Geometry: final body of the model. Coordinates: model frame, mm. A direction names the side the tool comes from. Round coordinates to 2 decimals unless told otherwise and drop trailing zeros. Write each loop counter-clockwise with the first axis right and the second up, starting at its lowest first coordinate (ties: lowest second). Pieces come first, ordered by that corner, then holes. Notation, with made-up numbers: (26, -7.75) -> (72, -7.75) arc R14 cw to (72, 1.25) -> close; hole circle Ø8 at (-6.5, 17). An arc over 180 degrees is marked (long way). One line per item, written item: value. Start each with the question number.
from build123d import *

# Parameters (mm, degrees)
SKETCH_1_W               = 56
SKETCH_1_H               = 30
EXTRUDE_1_DEPTH          = 8
SKETCH_3_W               = 32
SKETCH_3_H               = 30
EXTRUDE_2_DEPTH          = 4
EXTRUDE_3_DEPTH          = 12
EXTRUDE_4_DEPTH          = 8
CUT_EXTRUDE_1_DEPTH      = 46.803929962
CUT_EXTRUDE_1_DEPTH_BACK = 46.803929962


with BuildPart() as part:
    # Sketch 1 → Extrude 1 (new body)
    with BuildSketch(Plane(origin=(0, 0, 0), x_dir=(1, 0, 0), z_dir=(0, 1, 0))):
        Rectangle(SKETCH_1_W, SKETCH_1_H)
    extrude(amount=EXTRUDE_1_DEPTH)

    # Sketch 3 → Extrude 2 (add)
    with BuildSketch(Plane(origin=(0, 8, 0), x_dir=(1, 0, 0), z_dir=(0, 1, 0))):
        with Locations((-12, 0)):
            Rectangle(SKETCH_3_W, SKETCH_3_H)
    extrude(amount=EXTRUDE_2_DEPTH)

    # Sketch 7 → Extrude 3 (add)
    with BuildSketch(Plane.XY.offset(-15)):
        with BuildLine():
            Line((28, 8), (28, 21))
            ThreePointArc((28, 21), (16, 33), (4, 21))
            Line((4, 21), (4, 8))
            Line((4, 8), (28, 8))
        make_face()
        with BuildLine():
            ThreePointArc((10, 16), (16, 10), (22, 16))
            Line((22, 16), (22, 21))
            ThreePointArc((22, 21), (16, 27), (10, 21))
            Line((10, 21), (10, 16))
        make_face(mode=Mode.SUBTRACT)
    extrude(amount=EXTRUDE_3_DEPTH)

    # Sketch 7_4 → Extrude 4 (add)
    with BuildSketch(Plane.XY.offset(-15)):
        with BuildLine():
            Line((-28, 22.220866923), (-28, 12))
            Line((-28, 12), (4, 12))
            Line((4, 12), (4, 21))
            ThreePointArc((4, 21), (6.528997501, 28.368860948), (13.050018612, 32.631750075))
            Line((13.050018612, 32.631750075), (-28, 22.220866923))
        make_face()
    extrude(amount=EXTRUDE_4_DEPTH)

    # Sketch 13 → Cut-Extrude 1 (cut, two sides: drawn at the far end of the back side and taken through both)
    with BuildSketch(Plane(origin=(0, 0, 0), x_dir=(0, 0, -1), z_dir=(1, 0, 0)).offset(-CUT_EXTRUDE_1_DEPTH_BACK)):
        Polygon((0, 0), (6, 0), (8.886751346, 5), (-8.886751346, 5), (-6, 0), align=None)
    extrude(amount=CUT_EXTRUDE_1_DEPTH + CUT_EXTRUDE_1_DEPTH_BACK, mode=Mode.SUBTRACT)


solid = part.part
(1) Line query: probe 1 along Y at (x, z) = (9, 12); probe 2 along Y at (x, z) = (3.5, -2.25); probe 3 along Z at (x, y) = (-10.5, 17). Output: solid intervals per line, ascending.
(2) Set-up query: faces 5 (the face through (-12, 12, 4)), 6 (the face through (20.351, 32.183, -7.751)), 7 (the face through (10, 19, -9)), 8 (the face through (-7.19, 27.5, -11.06)), 9 (the face through (10, 23, -3)). Return all of +Z, -Z, +X, -X, +Y, -Y with unobstructed straight access to the full face (end or side cutting, diameter ignored); none if empty.
(3) Pull-direction query (Y, two-part tool) for faces 1 (the face through (-28, 9, -4)), 2 (the face through (16, 8, 6)), 3 (the face through (-0.392, 2.465, -7.423)), 4 (the face through (-0.39, 2.53, 7.46)); classes: pulls with the +Y half, pulls with the -Y half, needs draft (parallel to the pull), parting line crosses it, or undercut.
(4) Section query D-D (y = 30). Output: boundary loops of the cut face in (x, z), and give its area (3 significant figures).
(5) Section query C-C (x = -17.5). Output: boundary loops of the cut face in (y, z), and give its area (3 significant figures).
(6) Pin query (flat end, axial travel): pin 1 (6.5 mm diameter, centred on x = -19, z = 2.5, fed in from +Y); pin 2 (7 mm diameter, centred on x = 15, y = 17.5, fed in from +Z); pin 3 (2 mm diameter, centred on x = 13.5, z = 10.5, fed in from +Y); pin 4 (8 mm diameter, centred on y = 28.5, z = -11, fed in from +X). Return the tip coordinate at first contact, or that it passes through.
(7) Section query B-B (y = 15). Output: boundary loops of the cut face in (x, z).
(8) Section query A-A (x = 16). Output: boundary loops of the cut face in (y, z), and give its area (3 significant figures).
Results list:
1. probe 1: y = 0 to 8
1. probe 2: y = 5 to 12
1. probe 3: z = -15 to -7
2. face 5: +Z, -X, +Y
2. face 6: +Z, +Y
2. face 7: +Z, -Z
2. face 8: +Z, -Z, -X, +Y
2. face 9: +Z, +X, +Y
3. face 1: needs draft
3. face 2: pulls with the +Y half
3. face 3: undercut
3. face 4: undercut
4. outline: (2.67, -15) -> (23.94, -15) -> (23.94, -3) -> (8.06, -3) -> (8.06, -7) -> (2.67, -7) -> close
4. area: 234 mm^2
5. outline: (0, -15) -> (24.88, -15) -> (24.88, -7) -> (12, -7) -> (12, 15) -> (0, 15) -> (0, 6) -> (5, 8.89) -> (5, -8.89) -> (0, -6) -> close
5. area: 389 mm^2
6. pin 1: stops at y = 12
6. pin 2: passes through
6. pin 3: stops at y = 8
6. pin 4: stops at x = 27.48
7. outline: (-28, -15) -> (10.08, -15) -> (10.08, -3) -> (4, -3) -> (4, -7) -> (-28, -7) -> close; (21.92, -15) -> (28, -15) -> (28, -3) -> (21.92, -3) -> close
8. outline: (0, -15) -> (10, -15) -> (10, -3) -> (8, -3) -> (8, 15) -> (0, 15) -> (0, 6) -> (5, 8.89) -> (5, -8.89) -> (0, -6) -> close; (27, -15) -> (33, -15) -> (33, -3) -> (27, -3) -> close
8. area: 262 mm^2
